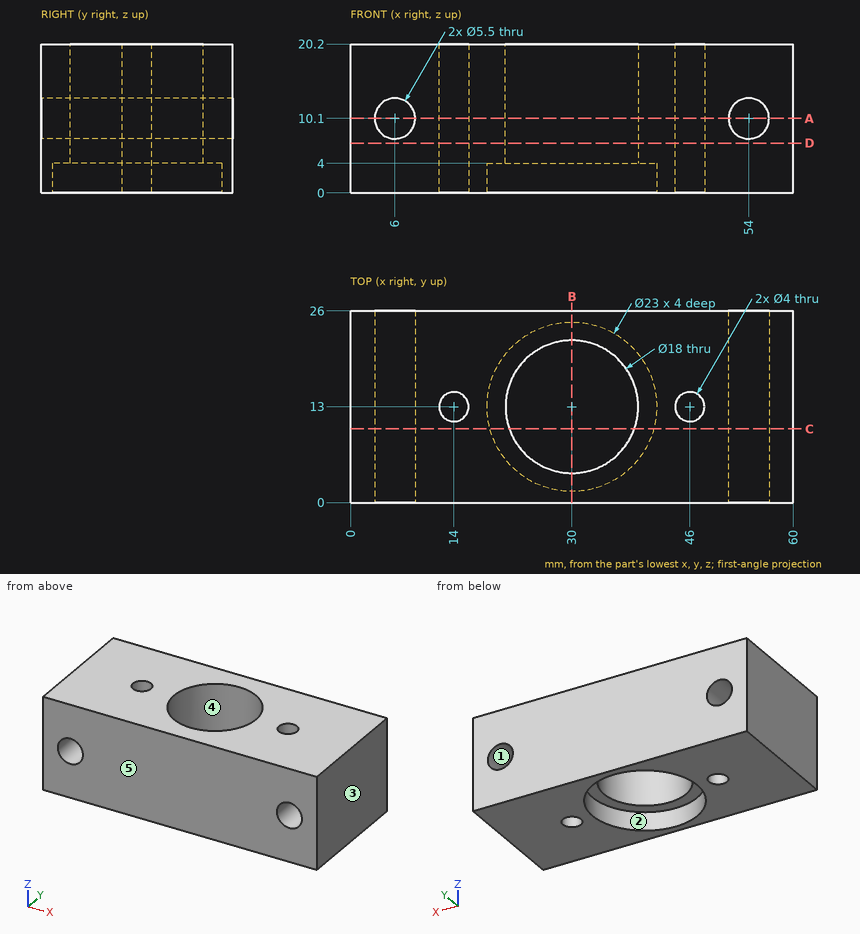
Study the drawing (mm; zero at the part's minimum x, y, z) and answer. A direction names the side the tool comes from. Coordinates: 2 decimals unless noted, no trailing zeros. Write each loop counter-clockwise with the first axis right and the second up, starting at its lowest first coordinate (ties: lowest second). Pieces come first, ordered by that corner, then holes. Notation, with made-up numbers: (-7, -33.75) - (48, -33.75) arc R10 ccw to (48, -16.75) - close; hole circle Ø7 at (73.5, 80). An arc over 180 degrees is marked (long way). Answer as a JSON object with one key per item and string values. Group by question number.
1. The mould has two halves that part along Y. Classify the marked faces 3, 4 and 5: +Y half, -Y half, draft (parallel to the pull), parting line (faces both ways), or undercut.
2. A cutting plane is placed at C-C (y = 10). Determine the outline of the cut face in (x, z).
3. Which of the six approach directions +Z, -Z, +X, -X, +Y, -Y give full straight-line access (tool end or side, diameter ignored) to the marked faces 1 and 2?
4. A cutting plane is placed at D-D (z = 6.75). Determine the outline of the cut face in (x, y).
5. A cutting plane is placed at B-B (x = 30). Determine the outline of the cut face in (y, z).
6. Consider L1, parallel to Y at x = 30, z = 2.3; L2, parallel to X at y = 9.5, z = 8.75; L3, parallel to Y at x = 14, z = 10.5. Determine where each line is inside the solid, lowest interval first. Write a range as [from, to].
7. A cutting plane is placed at A-A (z = 10.1). Determine the outline of the cut face in (x, y), plus the area to 3 significant figures.
8. Each of these flat-tipped pins is pushed along its axis until it touches: P1, Ø10, axis at y = 4.5, z = 6, coming from the -X side; P2, Ø11.5, axis at x = 33, y = 9, coming from the -Z side. Where does it stop, or does it pass through?
Worked out:
{
 "1": {"face 3": "draft", "face 4": "undercut", "face 5": "-Y half"},
 "2": {"outline": "(0, 0) - (18.9, 0) - (18.9, 4) - (21.51, 4) - (21.51, 20.2) - (0, 20.2) - close; (38.49, 4) - (41.1, 4) - (41.1, 0) - (60, 0) - (60, 20.2) - (38.49, 20.2) - close; hole circle Ø5.5 at (6, 10.1); hole circle Ø5.5 at (54, 10.1)"},
 "3": {"face 1": "+Y, -Y", "face 2": "-Z"},
 "4": {"outline": "(0, 0) - (60, 0) - (60, 26) - (0, 26) - close; hole circle Ø4 at (14, 13); hole circle Ø18 at (30, 13); hole circle Ø4 at (46, 13)"},
 "5": {"outline": "(0, 0) - (1.5, 0) - (1.5, 4) - (4, 4) - (4, 20.2) - (0, 20.2) - close; (22, 4) - (24.5, 4) - (24.5, 0) - (26, 0) - (26, 20.2) - (22, 20.2) - close"},
 "6": {"L1": "y = [0, 1.5], [24.5, 26]", "L2": "x = [0, 3.6], [8.4, 21.71], [38.29, 51.6], [56.4, 60]", "L3": "y = [0, 11], [15, 26]"},
 "7": {"outline": "(0, 0) - (3.25, 0) - (3.25, 26) - (0, 26) - close; (8.75, 0) - (51.25, 0) - (51.25, 26) - (8.75, 26) - close; (56.75, 0) - (60, 0) - (60, 26) - (56.75, 26) - close; hole circle Ø4 at (14, 13); hole circle Ø18 at (30, 13); hole circle Ø4 at (46, 13)", "area": "994 mm²"},
 "8": {"P1": "stops at x = 0", "P2": "stops at z = 4"}
}
